Input: dimensioned drawing with shaded views. Units: mm. Origin: part minimum x, y, z. Give positions to 0.01 mm unless a question says otherwise; leave off trailing zeros. Write each loop counter-clockwise with the first axis right and the second up, starting at its lowest first coordinate (ties: lowest second). Pieces come first, ordered by that corner, then holes.
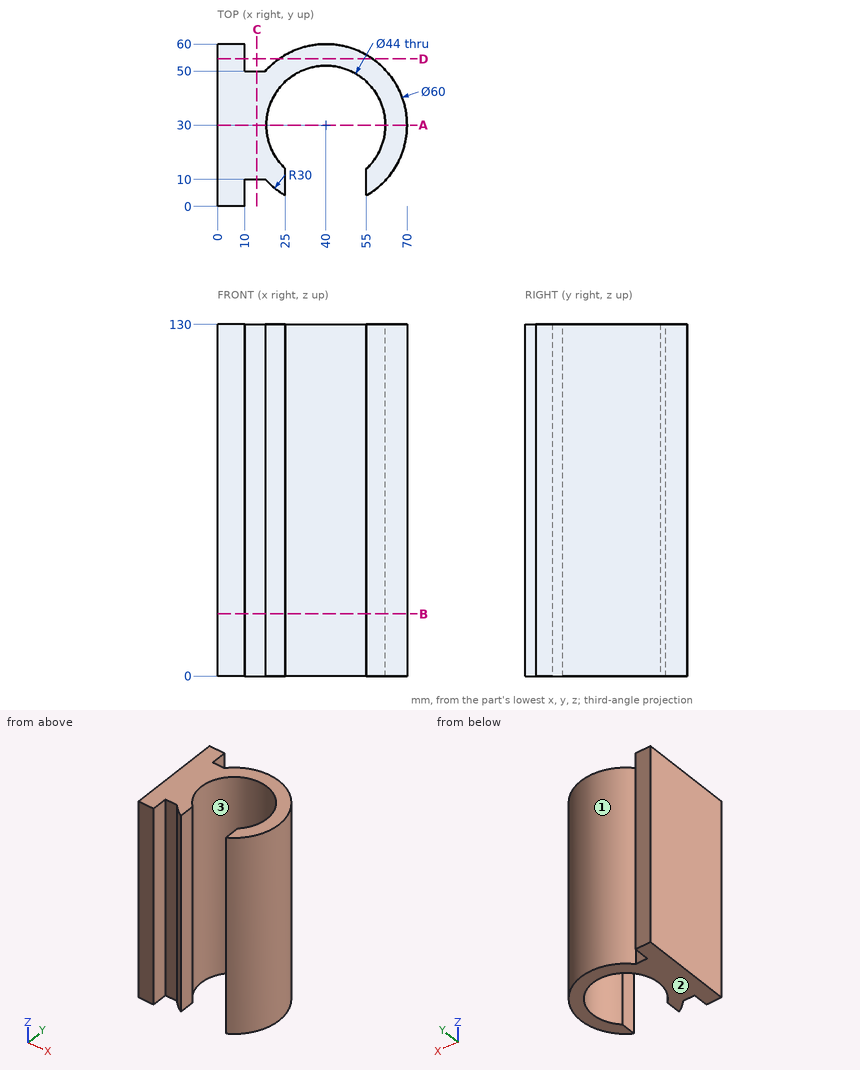
Item 1: Section C-C, the plane x = 14.5. Return the cut outline in (y, z).
Found:
outline: (10, 0) - (50, 0) - (50, 130) - (10, 130) - close
Item 2: Pull-direction query (Y, two-part tool) for the marked faces 1, 2 and 3; classes: +Y half, -Y half, draft (parallel to the pull), parting line (faces both ways), or undercut.
Found:
face 1: parting line
face 2: draft
face 3: undercut
Item 3: Section A-A, the plane y = 30. Return the cut outline in (x, z).
Found:
outline: (0, 0) - (18, 0) - (18, 130) - (0, 130) - close; (62, 0) - (70, 0) - (70, 130) - (62, 130) - close
Item 4: Section B-B, the plane z = 23. Return the cut outline in (x, y), plus the area to 3 significant figures.
Found:
outline: (0, 0) - (10, 0) - (10, 10) - (17.64, 10) arc R30 ccw to (25, 4.02) - (25, 13.91) arc R22 cw (long way) to (55, 13.91) - (55, 4.02) arc R30 ccw (long way) to (17.64, 50) - (10, 50) - (10, 60) - (0, 60) - close
area: 1,750 mm2
Item 5: Pin query (flat end, axial travel): pin 1 Ø3 at (y, z) = (9.5, 80) entering from +X; pin 2 Ø4 at (x, z) = (13.5, 61) entering from -Y; pin 3 Ø6 at (y, z) = (8.5, 81.5) entering from +X. Return the tip coordinate at first contact, or that it passes through.
Found:
pin 1: stops at x = 63.22
pin 2: stops at y = 10
pin 3: stops at x = 63.62
Item 6: Section D-D, the plane y = 54.5. Return the cut outline in (x, z).
Found:
outline: (0, 0) - (10, 0) - (10, 130) - (0, 130) - close; (22.69, 0) - (57.31, 0) - (57.31, 130) - (22.69, 130) - close
Item 7: Line query: L1, parallel to X at y = 6.5, z = 46; L2, parallel to X at y = 30, z = 43; L3, parallel to X at y = 37, z = 104. Output: solid intervals per line, ascending.
Found:
L1: x = 0 to 10, 21.35 to 25, 55 to 58.65
L2: x = 0 to 18, 62 to 70
L3: x = 0 to 19.14, 60.86 to 69.17
